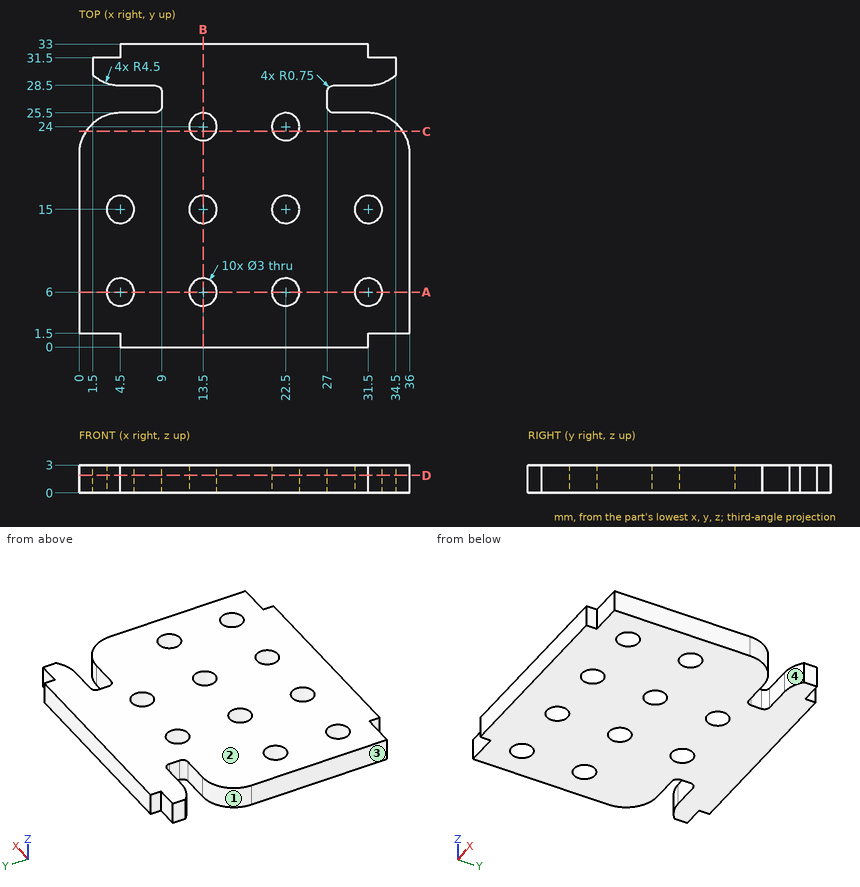
Job drawing, mm, ordinate dimensions from the low corner. One solid piece. A direction names the side the tool comes from. Coordinates: 2 decimals unless noted, no trailing zeros. Loops run counter-clockwise (first coordinate to the right, second up) from the corner with the lowest first, then second, coordinate; pieces in that order, holes last. Notation, with made-up numbers: (70, 65) - (86, 65) arc R24 ccw to (86, 75) - close; hole circle Ø5 at (79.25, 36.5). An arc over 180 degrees is marked (long way). Answer as a JSON object with one key per item and string values. Group by question number.
(1) Cut at D-D (z = 1.9). State how many separate pieces and enclosed holes the cut face has, then the cut area to 3 significant figures.
(2) Tool access for the marked faces 1 and 2: list every direction of +Z, -Z, +X, -X, +Y, -Y with a clear straight run to the whole face (end or side of a thin tool).
(3) Flat gauge pins, fed straight in: pin 1 (1.6 mm diameter, centred on y = 26.5, z = 1.5, fed in from -X); pin 2 (1.2 mm diameter, centred on y = 0.5, z = 2, fed in from +X); pin 3 (0.6 mm diameter, centred on y = 31, z = 1, fed in from +X). Where does each tip first touch, or does it go through?
(4) Cut at B-B (x = 13.5). Give the cut face in (y, z).
(5) Cut at C-C (y = 23.5). Give the cut face in (x, z).
(6) Cut at A-A (y = 6). Give the cut face in (x, z), then the cut area to 3 significant figures.
(7) Two-plate mould, pull along Y, no slides. Class the marked faces 3 and 4: released by +Y, released by -Y, zero draft, split by the parting line, or undercut.
(8) Probe line 1 along Y through (x, z) = (13.5, 1.7); line 2 along X through (y, z) = (6, 1.55); line 3 along X through (y, z) = (14, 0.9). List the from-to ranges inside material, lowest first.
Geometry says:
{
 "1": {"separate pieces": "1", "enclosed holes": "10", "area": "1,020 mm^2"},
 "2": {"face 1": "+Z, -Z, -X", "face 2": "+Z, +X, -X, +Y, -Y"},
 "3": {"pin 1": "stops at x = 8.76", "pin 2": "stops at x = 31.5", "pin 3": "stops at x = 34.5"},
 "4": {"outline": "(0, 0) - (4.5, 0) - (4.5, 3) - (0, 3) - close; (7.5, 0) - (13.5, 0) - (13.5, 3) - (7.5, 3) - close; (16.5, 0) - (22.5, 0) - (22.5, 3) - (16.5, 3) - close; (25.5, 0) - (33, 0) - (33, 3) - (25.5, 3) - close"},
 "5": {"outline": "(0.76, 0) - (12.09, 0) - (12.09, 3) - (0.76, 3) - close; (14.91, 0) - (21.09, 0) - (21.09, 3) - (14.91, 3) - close; (23.91, 0) - (35.24, 0) - (35.24, 3) - (23.91, 3) - close"},
 "6": {"outline": "(0, 0) - (3, 0) - (3, 3) - (0, 3) - close; (6, 0) - (12, 0) - (12, 3) - (6, 3) - close; (15, 0) - (21, 0) - (21, 3) - (15, 3) - close; (24, 0) - (30, 0) - (30, 3) - (24, 3) - close; (33, 0) - (36, 0) - (36, 3) - (33, 3) - close", "area": "72.0 mm^2"},
 "7": {"face 3": "zero draft", "face 4": "undercut"},
 "8": {"line 1": "y = 0 to 4.5, 7.5 to 13.5, 16.5 to 22.5, 25.5 to 33", "line 2": "x = 0 to 3, 6 to 12, 15 to 21, 24 to 30, 33 to 36", "line 3": "x = 0 to 3.38, 5.62 to 12.38, 14.62 to 21.38, 23.62 to 30.38, 32.62 to 36"}
}
